```python
from build123d import *

# Parameters (mm, degrees)
SKETCH1_R           = 4.7625
BOSS_EXTRUDE1_DEPTH = 31.75
SKETCH2_R           = 6.35
BOSS_EXTRUDE2_DEPTH = 6.35
CHAMFER1_SIZE       = 2.38
SKETCH3_R           = 3.175
CUT_EXTRUDE1_DEPTH  = 12.7
BOSS_EXTRUDE3_START = 31.75
SKETCH4_R           = 4.7625
BOSS_EXTRUDE3_DEPTH = 31.75
BOSS_EXTRUDE4_START = 6.35
SKETCH5_R           = 6.35
BOSS_EXTRUDE4_DEPTH = 6.35
CHAMFER2_SIZE       = 2.38
CUT_EXTRUDE2_START  = -12.7
SKETCH6_R           = 3.175
CUT_EXTRUDE2_DEPTH  = 12.7


with BuildPart() as part:
    # Sketch1 → Boss-Extrude1 (new body)
    with BuildSketch(Plane.XY):
        Circle(SKETCH1_R)
    extrude(amount=BOSS_EXTRUDE1_DEPTH)

    # Sketch2 → Boss-Extrude2 (add)
    with BuildSketch(Plane.XY.offset(31.75)):
        Circle(SKETCH2_R)
    extrude(amount=BOSS_EXTRUDE2_DEPTH)

    # Chamfer1
    # the kernel refuses this chamfer: 2.38 mm, written as the material it takes off along each edge
    with BuildSketch(Plane(origin=(0, 0, 31.75), x_dir=(1, 0, 0), z_dir=(0, -1, 0))) as chamfer1_piece_1_section:
        Polygon((6.35, CHAMFER1_SIZE), (6.35 - CHAMFER1_SIZE, 0), (6.35, 0), align=None)
    chamfer1_piece_1 = revolve(axis=Axis((0, 0, 31.75), (0, 0, 1)), mode=Mode.PRIVATE)
    chamfer1_piece_1 = chamfer1_piece_1 - Plane(origin=(0, 0, 33.337286279), x_dir=(1, 0, 0), z_dir=(0, 0, -1)) * Cylinder(4.7625, 26, mode=Mode.PRIVATE)
    add(chamfer1_piece_1, mode=Mode.SUBTRACT)

    # Sketch3 → Cut-Extrude1 (cut)
    with BuildSketch(Plane.XY.offset(38.1)):
        Circle(SKETCH3_R)
    extrude(amount=-CUT_EXTRUDE1_DEPTH, mode=Mode.SUBTRACT)

    # Sketch4 → Boss-Extrude3 (add)
    with BuildSketch(Plane(origin=(0, 0, 0), x_dir=(-1, 0, 0), z_dir=(0, 0, -1)).offset(BOSS_EXTRUDE3_START)):
        Circle(SKETCH4_R)
    extrude(amount=-BOSS_EXTRUDE3_DEPTH)

    # Sketch5 → Boss-Extrude4 (add)
    with BuildSketch(Plane(origin=(0, 0, -31.75), x_dir=(-1, 0, 0), z_dir=(0, 0, -1)).offset(BOSS_EXTRUDE4_START)):
        with Locations(Location((0, 0, 0), (0, 0, 180))):
            Circle(SKETCH5_R)
    extrude(amount=-BOSS_EXTRUDE4_DEPTH)

    # Chamfer2
    # the kernel refuses this chamfer: 2.38 mm, written as the material it takes off along each edge
    with BuildSketch(Plane(origin=(0, 0, -31.75), x_dir=(1, 0, 0), z_dir=(0, 1, 0))) as chamfer2_piece_1_section:
        Polygon((6.35, CHAMFER2_SIZE), (6.35 - CHAMFER2_SIZE, 0), (6.35, 0), align=None)
    chamfer2_piece_1 = revolve(axis=Axis((0, 0, -31.75), (0, 0, -1)), mode=Mode.PRIVATE)
    chamfer2_piece_1 = chamfer2_piece_1 - Plane(origin=(0, 0, -33.337286279), x_dir=(-1, 0, 0), z_dir=(0, 0, -1)) * Cylinder(4.7625, 26, mode=Mode.PRIVATE)
    add(chamfer2_piece_1, mode=Mode.SUBTRACT)

    # Sketch6 → Cut-Extrude2 (cut)
    with BuildSketch(Plane(origin=(0, 0, -38.1), x_dir=(-1, 0, 0), z_dir=(0, 0, -1)).offset(CUT_EXTRUDE2_START)):
        with Locations(Location((0, 0, 0), (0, 0, 180))):
            Circle(SKETCH6_R)
    extrude(amount=CUT_EXTRUDE2_DEPTH, mode=Mode.SUBTRACT)


solid = part.part
```
Part model, mm, in its own coordinate system. A direction names the side the tool comes from. Coordinates: 2 decimals unless noted, no trailing zeros. Loops run counter-clockwise (first coordinate to the right, second up) from the corner with the lowest first, then second, coordinate; pieces in that order, holes last. Notation, with made-up numbers: (-22.5, 10.25) - (1.5, 10.25) arc R22 ccw to (1.5, 17.25) - close; hole circle Ø5 at (-21, 16). An arc over 180 degrees is marked (long way). Write item = value, one per line. Start each with the question number.
Item 1: Mould opens along Z. For faces 3 (the flat face through (0, 0, -25.4)), 4 (the cylindrical face through (1.5, 2.8, -31.7)), 5 (the flat face through (-2, 3, 38.1)) say: released by +Z, released by -Z, zero draft, split by the parting line, or undercut.
Item 2: Wall check: L1, parallel to Y at x = 0, z = 28.75 (1 decimal); L2, parallel to Y at x = 0, z = 35 (3 decimals); L3, parallel to Z at x = 1.75, y = -1.5. Give the ranges that are in metal, low to high. Write a range as from..to.
Item 3: Flat gauge pins, fed straight in: pin 1 Ø5 at (x, y) = (0, 0) entering from -Z; pin 2 Ø3 at (x, y) = (-1.5, 0.5) entering from +Z; pin 3 Ø4 at (x, z) = (-4.5, 5.5) entering from +Y. Where does each tip first touch, or does it go through?
Item 4: Cut at C-C, the plane z = -19. Give the cut face in (x, y) (1 decimal), and give its area (3 significant figures).
Item 5: 3-axis set-ups, long thin cutter, end or side, ignore diameter. For faces 1 (the cylindrical face through (2.93, 5.634, -36.143)), 2 (the flat face through (0, 0, 25.4)): which of +Z, -Z, +X, -X, +Y, -Y reach the whole face in a straight line?
The answers:
q1.face_3 = released by -Z
q1.face_4 = zero draft
q1.face_5 = released by +Z
q2.L1 = -4.8..-3.2, 3.2..4.8
q2.L2 = -6.35..-3.175, 3.175..6.35
q2.L3 = -25.4..25.4
q3.pin_1 = -25.4
q3.pin_2 = 25.4
q3.pin_3 = 4.05
q4.outline = circle Ø9.5 at (0, 0)
q4.area = 71.3 mm2
q5.face_1 = +Z, -Z
q5.face_2 = +Z
